```python
from build123d import *

# Parameters (mm, degrees)
SKETCH1_W           = 84
SKETCH1_H           = 34.5
BOSS_EXTRUDE1_DEPTH = 6.8
SKETCH2_W           = 64.5
SKETCH2_H           = 34.5
BOSS_EXTRUDE2_DEPTH = 19.6
SKETCH3_R           = 1.75
CUT_EXTRUDE1_DEPTH  = 6.8
FILLET1_R           = 1
FILLET2_R           = 1


with BuildPart() as part:
    # Sketch1 → Boss-Extrude1 (new body)
    with BuildSketch(Plane(origin=(0, 0, 0), x_dir=(1, 0, 0), z_dir=(0, 1, 0))):
        with Locations((25.748743719, -8.498743719)):
            Rectangle(SKETCH1_W, SKETCH1_H)
    extrude(amount=BOSS_EXTRUDE1_DEPTH)

    # Sketch2 → Boss-Extrude2 (add)
    with BuildSketch(Plane(origin=(0, 6.8, 0), x_dir=(1, 0, 0), z_dir=(0, 1, 0))):
        with Locations((25.824659205, -8.498743719)):
            Rectangle(SKETCH2_W, SKETCH2_H)
    extrude(amount=BOSS_EXTRUDE2_DEPTH)

    # Sketch3 → Cut-Extrude1 (cut)
    with BuildSketch(Plane(origin=(0, 6.8, 0), x_dir=(1, 0, 0), z_dir=(0, 1, 0))):
        with Locations(Location((63.248743719, 4.201256281, 0), (0, 0, 270))):
            Circle(SKETCH3_R)
        with Locations(Location((63.248743719, -21.198743719, 0), (0, 0, 270))):
            Circle(SKETCH3_R)
        with Locations(Location((-11.751256281, -21.198743719, 0), (0, 0, 270))):
            Circle(SKETCH3_R)
        with Locations(Location((-11.751256281, 4.201256281, 0), (0, 0, 270))):
            Circle(SKETCH3_R)
    extrude(amount=-CUT_EXTRUDE1_DEPTH, mode=Mode.SUBTRACT)

    # Fillet1
    fillet1_edges = [part.edges().sort_by_distance(p)[0] for p in [
        (-16.251256281, 3.4, -8.751256281),
        (67.748743719, 3.4, -8.751256281),
        (67.748743719, 3.4, 25.748743719),
        (-16.251256281, 3.4, 25.748743719),
    ]]
    fillet(fillet1_edges, radius=FILLET1_R)

    # Fillet2
    fillet2_edges = [part.edges().sort_by_distance(p)[0] for p in [
        (-6.425340795, 16.6, -8.751256281),
        (-6.425340795, 16.6, 25.748743719),
        (58.074659205, 16.6, 25.748743719),
        (58.074659205, 16.6, -8.751256281),
    ]]
    fillet(fillet2_edges, radius=FILLET2_R)


solid = part.part
```
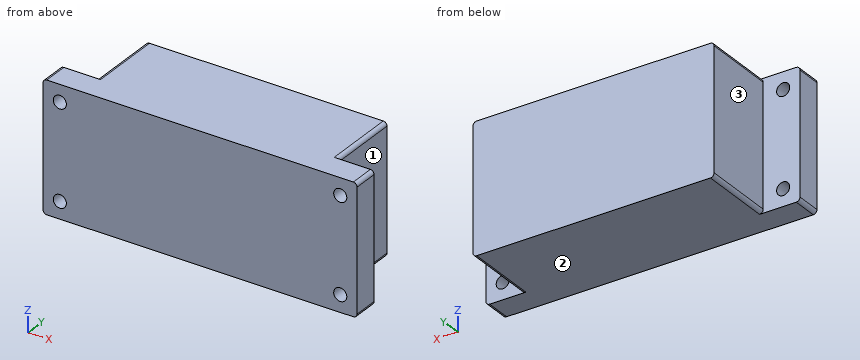
Read the model definition and answer for the solid it produces. Units are mm, in the model's axes. Face numbers are marked on the shaded views. A direction names the side the tool comes from. Give positions to 0.01 mm unless a question says otherwise; leave off trailing zeros. Write each loop counter-clockwise with the first axis right and the second up, starting at its lowest first coordinate (ties: lowest second). Pieces come first, ordered by that corner, then holes. Notation, with made-up numbers: M 32,82.5 L 39,82.5 A33 cw 39,113.5 Z; hole C 13,28 d3. An arc over 180 degrees is marked long. Put each result on its own line as item: value. Start each with the question number.
1. Which of the six approach directions +Z, -Z, +X, -X, +Y, -Y give full straight-line access (tool end or side, diameter ignored) to the marked faces 1, 2 and 3?
2. The part is cut by section C-C, the plane z = 22. Give the vertices of the cut face in (x, y), and give its area (3 significant figures).
3. The part is cut by section A-A, the plane z = 2.5. Give the vertices of the cut face in (x, y).
4. The part is cut by section B-B, the plane y = 9. Give the vertices of the cut face in (x, z), and give its area (3 significant figures).
5. Consider line 1 along Z through (x, y) = (-11.5, 4); line 2 along X through (y, z) = (7, 7.5); line 3 along Y through (x, z) = (-8, 17). Determine where each line is inside the solid, lowest interval first.
6. Each of these flat-tipped pins is pushed along its axis until it touches: pin 1 Ø4 at (x, z) = (-11.75, 21.2) entering from +Y; pin 2 Ø3 at (y, z) = (15, 6) entering from -X; pin 3 Ø12 at (x, z) = (-12, 5.5) entering from +Y; pin 4 Ø1.5 at (y, z) = (14.5, 15) entering from +X. Where does it stop, or does it pass through?
Final values:
1. face 1: +Z, -Z, +X, +Y
1. face 2: -Z, +X, -X, +Y, -Y
1. face 3: +Z, -Z, -X, +Y
2. outline: M -16.25,0 L -13.31,0 L -13.31,6.8 L -16.25,6.8 Z; M -10.2,0 L 61.69,0 L 61.69,6.8 L 58.07,6.8 L 58.07,26.4 L -6.43,26.4 L -6.43,6.8 L -10.2,6.8 Z; M 64.8,0 L 67.75,0 L 67.75,6.8 L 64.8,6.8 Z
2. area: 1,790 mm²
3. outline: M -16.25,0 L 67.75,0 L 67.75,6.8 L 58.07,6.8 L 58.07,26.4 L -6.43,26.4 L -6.43,6.8 L -16.25,6.8 Z
4. outline: M -6.43,-7.75 A1 ccw -5.43,-8.75 L 57.07,-8.75 A1 ccw 58.07,-7.75 L 58.07,24.75 A1 ccw 57.07,25.75 L -5.43,25.75 A1 ccw -6.43,24.75 Z
4. area: 2,220 mm²
5. line 1: z = -8.75 to -5.93, -2.47 to 19.47, 22.93 to 25.75
5. line 2: x = -6.43 to 58.07
5. line 3: y = 0 to 6.8
6. pin 1: stops at y = 6.8
6. pin 2: stops at x = -6.43
6. pin 3: stops at y = 26.4
6. pin 4: stops at x = 58.07
